```python
from build123d import *

# Parameters (mm, degrees)
F0_R     = 5.75
F1_DEPTH = 70
F4_DEPTH = 25
F6_R     = 8
F7_DEPTH = 2


with BuildPart() as f1:
    # F0 (on Right) → F1 (new body)
    with BuildSketch(Plane.YZ):
        Circle(F0_R)
    extrude(amount=F1_DEPTH)

    # F3 (on offset) → F4 (cut)
    with BuildSketch(Plane.XY.offset(6.8)):
        with BuildLine():
            Line((11.25, 0), (13, 0))
            Line((13, 0), (14.75, 0))
            ThreePointArc((14.75, 0), (13, 1.75), (11.25, 0))
        make_face()
        with BuildLine():
            Line((14.75, 0), (13, 0))
            Line((13, 0), (11.25, 0))
            ThreePointArc((11.25, 0), (13, -1.75), (14.75, 0))
        make_face()
    extrude(amount=-F4_DEPTH, mode=Mode.SUBTRACT)

    # F6 (on offset) → F7 (join)
    with BuildSketch(Plane.YZ.offset(55)):
        Circle(F6_R)
    extrude(amount=F7_DEPTH)


solid = f1.part
```
Here's how the part is built. I have some questions about the finished solid (model axes, mm). A direction names the side the tool comes from. Coordinates: 2 decimals unless noted, no trailing zeros. Write each loop counter-clockwise with the first axis right and the second up, starting at its lowest first coordinate (ties: lowest second). Pieces come first, ordered by that corner, then holes. Notation, with made-up numbers: (89, -37.75) - (130, -37.75) arc R12 ccw to (130, -31.75) - close; hole circle Ø4 at (59, 18). An arc over 180 degrees is marked (long way). One line per item, written item: value.
1) On a 3-axis mill with a long thin cutter (end or side, diameter ignored), from which of +Z, -Z, +X, -X, +Y, -Y can I reach the whole of each face in a straight line? I mean faces 4 (the flat face through (70, 0, 0)), 5 (the flat face through (57, 5.2, -3.4)), 6 (the cylindrical face through (27.12, -0.75, 5.7)). Say none if no direction works.
Model answer:
face 4: +Z, -Z, +X, +Y, -Y
face 5: +X
face 6: -X
2) I'm going to push flat-ended pins straight in: P1, Ø4, axis at x = 53.5, y = -3, coming from the +Z side; P2, Ø3, axis at x = 23, z = 2, coming from the +Y side; P3, Ø3, axis at x = 30.5, y = -2, coming from the +Z side. Where does each tip first touch, or does it pass through?
Model answer:
P1: stops at z = 7.82
P2: stops at y = 5.73
P3: stops at z = 5.73
3) Suppose I cut it at D-D on z = -4.25. Write out the boundary of the cut face in (x, y), and give its area (3 significant figures).
Model answer:
outline: (0, -3.87) - (55, -3.87) - (55, -6.78) - (57, -6.78) - (57, -3.87) - (70, -3.87) - (70, 3.87) - (57, 3.87) - (57, 6.78) - (55, 6.78) - (55, 3.87) - (0, 3.87) - close; hole circle Ø3.5 at (13, 0)
area: 544 mm²
4) I need wall thicknesses on line 1 along X through (y, z) = (0, -2.75); line 2 along Y through (x, z) = (13, 0); line 3 along X through (y, z) = (5.75, 4.25). Which ranges of each line are inside material? Lowest first, please.
Model answer:
line 1: x = 0 to 11.25, 14.75 to 70
line 2: y = -5.75 to -1.75, 1.75 to 5.75
line 3: x = 55 to 57
5) Suppose I cut it at B-B on y = 0. Write out the boundary of the cut face in (x, z).
Model answer:
outline: (0, -5.75) - (11.25, -5.75) - (11.25, 5.75) - (0, 5.75) - close; (14.75, -5.75) - (55, -5.75) - (55, -8) - (57, -8) - (57, -5.75) - (70, -5.75) - (70, 5.75) - (57, 5.75) - (57, 8) - (55, 8) - (55, 5.75) - (14.75, 5.75) - close
6) Suppose I cut it at A-A on z = 0. Write out the boundary of the cut face in (x, y).
Model answer:
outline: (0, -5.75) - (55, -5.75) - (55, -8) - (57, -8) - (57, -5.75) - (70, -5.75) - (70, 5.75) - (57, 5.75) - (57, 8) - (55, 8) - (55, 5.75) - (0, 5.75) - close; hole circle Ø3.5 at (13, 0)
7) We'd pull the mould along Y, two halves only. Please class faces 1 (the cylindrical face through (11.331, -0.526, 0.081)), 2 (the flat face through (55, 5.2, -3.4)), 3 (the cylindrical face through (63.41, -0.75, 5.7)): pulls with the +Y half, pulls with the -Y half, needs draft (parallel to the pull), parting line crosses it, or undercut.
Model answer:
face 1: undercut
face 2: needs draft
face 3: parting line crosses it
8) Suppose I cut it at C-C on y = 4.75. Write out the boundary of the cut face in (x, z), and give its area (3 significant figures).
Model answer:
outline: (0, -3.24) - (55, -3.24) - (55, -6.44) - (57, -6.44) - (57, -3.24) - (70, -3.24) - (70, 3.24) - (57, 3.24) - (57, 6.44) - (55, 6.44) - (55, 3.24) - (0, 3.24) - close
area: 466 mm²
